The listing builds one solid part. Answer for the finished solid, in the listing's coordinates (mm). Round coordinates to 2 decimals unless told otherwise and drop trailing zeros. Loops run counter-clockwise (first coordinate to the right, second up) from the corner with the lowest first, then second, coordinate; pieces in that order, holes last. Notation, with made-up numbers: M 23.25,33 L 68.25,33 A35 ccw 68.25,72 Z; hole C 4.25,-29 d1. An arc over 180 degrees is marked long. Answer as a JSON object with one key per item and string values.
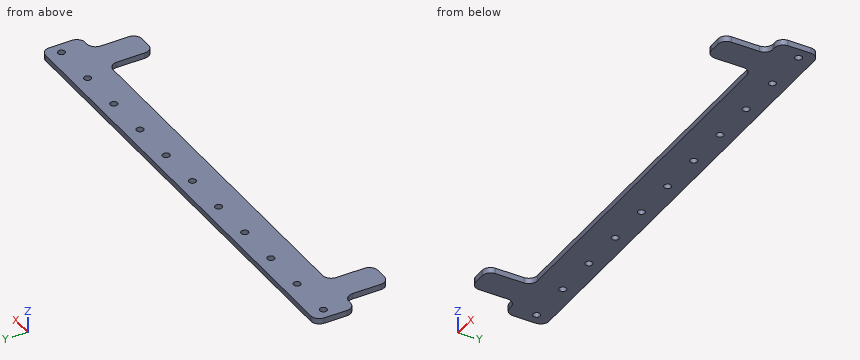
```python
from build123d import *

# Parameters (mm, degrees)
BASE_SKETCH_W            = 168
BASE_SKETCH_H            = 14
BASE_EXTRUDE_DEPTH       = 2
PIN_HOLE_SKETCH_R        = 1.25
FIRST_PIN_HOLE_CUT_DEPTH = 85.314885993
PIN_HOLE_PATTERN_COUNT   = 11
PIN_HOLE_PATTERN_PITCH   = 16
EXTENSION_SKETCH_W       = 10
EXTENSION_SKETCH_H       = 25
TAB_EXTRUDE_DEPTH        = 2
CORNER_FILLETS_R         = 3


with BuildPart() as part:
    # Base Sketch → Base Extrude (new body)
    with BuildSketch(Plane.XY):
        Rectangle(BASE_SKETCH_W, BASE_SKETCH_H)
    extrude(amount=-BASE_EXTRUDE_DEPTH)

    # Pin Hole Sketch → First Pin Hole Cut (cut, through all)
    with BuildSketch(Plane.XY):
        with Locations((80, 2)):
            Circle(PIN_HOLE_SKETCH_R)
    first_pin_hole_cut = extrude(amount=-FIRST_PIN_HOLE_CUT_DEPTH, mode=Mode.SUBTRACT)

    # Pin Hole Pattern: First Pin Hole Cut ×11
    with Locations(*[(-i * PIN_HOLE_PATTERN_PITCH, 0, 0) for i in range(1, PIN_HOLE_PATTERN_COUNT)]):
        add(first_pin_hole_cut, mode=Mode.SUBTRACT)


with BuildPart() as body_2:
    # Extension Sketch → Tab Extrude (new, through all)
    with BuildSketch(Plane.XY):
        with Locations((72, -10.5)):
            Rectangle(EXTENSION_SKETCH_W, EXTENSION_SKETCH_H)
    tab_extrude = extrude(amount=-TAB_EXTRUDE_DEPTH)


with BuildPart() as part_1:
    add(part.part)

    # Tab Mirror: Tab Extrude across plane
    add(tab_extrude.mirror(Plane(origin=(0, 0, 0), x_dir=(0, 0, 1), z_dir=(1, 0, 0))))

    # Combine Bodies: union body 2
    add(body_2.part)

    # Corner Fillets
    corner_fillets_edges = [part_1.edges().sort_by_distance(p)[0] for p in [
        (-77, -7, -1),
        (-77, -23, -1),
        (-67, -23, -1),
        (-67, -7, -1),
        (77, -7, -1),
        (77, -23, -1),
        (67, -7, -1),
        (67, -23, -1),
        (-84, 7, -1),
        (84, 7, -1),
        (84, -7, -1),
        (-84, -7, -1),
    ]]
    fillet(corner_fillets_edges, radius=CORNER_FILLETS_R)


solid = part_1.part
```
Item 1: Straight lines are drawn through the part: line 1 (X direction, y = -15.5, z = -1.9); line 2 (Y direction, x = -48, z = -0.4); line 3 (Y direction, x = 3, z = -0.1). For each, find the intervals that lie inside material, in ascending order.
Values follow:
{"line 1": "-77 to -67, 67 to 77", "line 2": "-7 to 0.75, 3.25 to 7", "line 3": "-7 to 7"}
Item 2: The part is cut by section B-B (z = -0.9). Give the number of separate pieces and of enclosed holes in the cut face, then the cut area to 3 significant figures.
Values follow:
{"separate pieces": "1", "enclosed holes": "11", "area": "2,610 mm^2"}
Item 3: The part is cut by section A-A (y = -17.5). Give the vertices of the cut face in (x, z).
Values follow:
{"outline": "M -77,-2 L -67,-2 L -67,0 L -77,0 Z; M 67,-2 L 77,-2 L 77,0 L 67,0 Z"}
Item 4: Flat-ended cylindrical pins translate along their axes: P1, Ø1, axis at x = 2, z = -1, coming from the -Y side; P2, Ø2, axis at x = 64, y = 2, coming from the -Z side; P3, Ø0.6, axis at y = -14.5, z = -0.5, coming from the +X side; P4, Ø3, axis at x = 80, y = 2, coming from the +Z side. Find the tip coordinate at first contact, or state that the pin passes through.
Values follow:
{"P1": "y = -7", "P2": "through", "P3": "x = 77", "P4": "z = 0"}
Item 5: The part is cut by section C-C (x = 8.5). Give the vertices of the cut face in (y, z), then the cut area to 3 significant figures.
Values follow:
{"outline": "M -7,-2 L 7,-2 L 7,0 L -7,0 Z", "area": "28.0 mm^2"}
